The listing builds one solid part. Answer for the finished solid, in the listing's coordinates (mm). Face numbers are marked on the shaded views. A direction names the side the tool comes from. Coordinates: 2 decimals unless noted, no trailing zeros. Write each loop counter-clockwise with the first axis right and the second up, starting at its lowest first coordinate (ties: lowest second). Pieces come first, ordered by that corner, then holes.
(1) The part is cut by section B-B on x = 2.75. Determine the outline of the cut face in (y, z).
(2) Which of the six approach directions +Z, -Z, +X, -X, +Y, -Y give full straight-line access (tool end or side, diameter ignored) to the marked faces 1 and 2?
(3) The part is cut by section D-D on z = 9.5. Determine the outline of the cut face in (x, y).
(4) The part is cut by section C-C on x = 11.25. Determine the outline of the cut face in (y, z).
(5) Given P1, Ø6, axis at x = 3, y = 3, coming from the +Z side; P2, Ø6, axis at x = 2.5, z = 21.5, coming from the +Y side; P3, Ø3, axis at x = 6.5, y = 47, coming from the +Z side; P4, Ø3, axis at y = 11, z = 22, coming from the +X side, each flat-ended and moving along its own axis, determine where each tip first touches the part or whether it passes through.
(6) For a pull along Y with two mould halves and no side action, classify the marked faces 3, 4, 5 and 6 as +Y half, -Y half, draft (parallel to the pull), parting line (faces both ways), or undercut.
(7) The part is cut by section A-A on y = 68.5. Determine the outline of the cut face in (x, z), plus the area to 3 significant figures.
(8) Straight lines are drawn through the part: line 1 (Y direction, x = 3, z = 4.75); line 2 (X direction, y = 68.5, z = 5.25); line 3 (Y direction, x = 3, z = 2.75). For each, find the intervals that lie inside material, in ascending order.
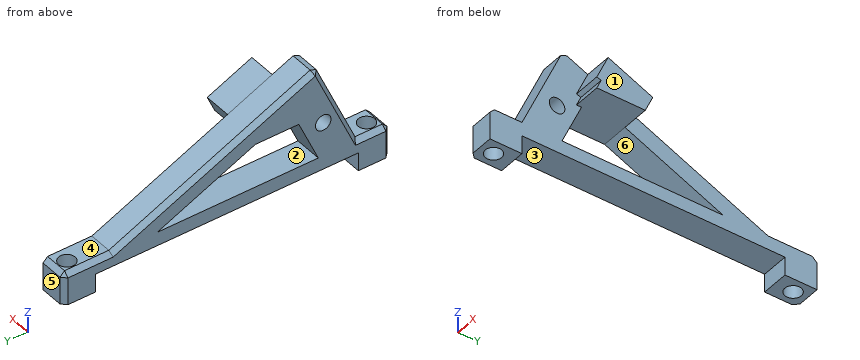
from build123d import *

# Parameters (mm, degrees)
SKETCH006_R     = 1.7
PAD003_DEPTH    = 6
SKETCH007_R     = 1.8
POCKET003_DEPTH = 7
PAD004_DEPTH    = 12
CHAMFER002_SIZE = 1


with BuildPart() as support:
    # Sketch006 → Pad003 (new body)
    with BuildSketch(Plane.YZ):
        Polygon((71.5, 0), (71.5, -7), (60.825309, -7), (15.904574, -27), (7, -7), (0, -7), (0, 0), (7, 0), (7, -4), (64.5, -4), (64.5, 0), align=None)
        with Locations((14.677916, -14.410508)):
            Circle(SKETCH006_R, mode=Mode.SUBTRACT)
        Polygon((15.75709, -7), (50.990936, -7), (21.585991, -20.091925), align=None, mode=Mode.SUBTRACT)
    extrude(amount=PAD003_DEPTH)

    # Sketch007 → Pocket003 (cut)
    with BuildSketch(Plane.XY):
        with Locations((3, 68.5)):
            Circle(SKETCH007_R)
        with Locations((3, 3)):
            Circle(SKETCH007_R)
    extrude(amount=-POCKET003_DEPTH, mode=Mode.SUBTRACT)

    # Sketch008 → Pad004 (join)
    with BuildSketch(Plane.YZ):
        Polygon((21.385846, -24.55958), (18.945427, -19.078307), (19.858972, -18.671571), (18.918653, -16.55958), (29.519767, -16.55958), (31.146714, -20.213762), align=None)
    extrude(amount=PAD004_DEPTH)

    # Chamfer002
    chamfer002_edges = [support.edges().sort_by_distance(p)[0] for p in [
        (0, 66.162655, -7),
        (0, 45.986012, -13.606881),
        (0, 26.26628, -22.386671),
        (0, 18.64521, -25.77979),
        (0, 11.452287, -17),
        (0, 3.5, -7),
        (3, 0, -7),
        (3, 15.904574, -27),
        (3, 71.5, -7),
        (0, 0, -3.5),
        (0, 71.5, -3.5),
    ]]
    chamfer(chamfer002_edges, length=CHAMFER002_SIZE)


with BuildPart() as support_mirror:
    # Part__Mirroring: instance of support
    add(support.part.mirror(Plane(origin=(0, 0, 0), x_dir=(0, 1, 0), z_dir=(0, 0, 1))))


solid = support_mirror.part
Model answer:
1. outline: (0, 0) - (1.22, 0) - (1.22, 7) - (1, 7) - (0, 6) - close; (4.78, 0) - (7, 0) - (7, 4) - (64.5, 4) - (64.5, 0) - (66.72, 0) - (66.72, 7) - (60.83, 7) - (16.82, 26.59) - (15.5, 26.09) - (7, 7) - (4.78, 7) - close; (70.28, 0) - (71.5, 0) - (71.5, 6) - (70.5, 7) - (70.28, 7) - close; hole circle Ø3.4 at (14.68, 14.41); hole (15.76, 7) - (50.99, 7) - (29.52, 16.56) - (20.01, 16.56) - close
2. face 1: +Z, -Z, +X, +Y, -Y
2. face 2: +X, -X
3. outline: (0, 9.21) - (1, 8.11) - (6, 8.11) - (6, 16.87) - (0, 16.87) - close; (0, 45.38) - (6, 45.38) - (6, 55.21) - (1, 55.21) - (0, 52.75) - close
4. outline: (18.92, 16.56) - (29.52, 16.56) - (31.15, 20.21) - (21.39, 24.56) - (18.95, 19.08) - (19.86, 18.67) - close
5. P1: stops at z = 7
5. P2: stops at y = 35
5. P3: stops at z = 13.79
5. P4: passes through
6. face 3: undercut
6. face 4: draft
6. face 5: +Y half
6. face 6: undercut
7. outline: (0, 0) - (1.2, 0) - (1.2, 7) - (1, 7) - (0, 6) - close; (4.8, 0) - (6, 0) - (6, 7) - (4.8, 7) - close
7. area: 16.3 mm2
8. line 1: y = 0 to 1.2, 4.8 to 66.7, 70.3 to 71.5
8. line 2: x = 0 to 1.2, 4.8 to 6
8. line 3: y = 0 to 1.2, 4.8 to 7, 64.5 to 66.7, 70.3 to 71.5
